Autodesk Inventor part; units mm, degrees
ref_plane "YZ Plane" through (0, 0, 0) normal (1, 0, 0) x (0, 1, 0)
ref_plane "XZ Plane" through (0, 0, 0) normal (0, 1, 0) x (-1, 0, 0)
ref_plane "XY Plane" through (0, 0, 0) normal (0, 0, 1) x (1, 0, 0)
sketch "Sketch1" plane through (0, 0, 0) normal (0, 1, 0) x (-1, 0, 0)
  circle A0 centre (0, 0) radius 6.985
  line L0 (6.985, 0) -> (6.985, -21.59)
  line L1 (6.985, -21.59) -> (-6.985, -21.59)
  line L2 (-6.985, -21.59) -> (-6.985, 0)
  line L3 (0, 0) -> (1.651, 0)
  line L4 (1.651, 0) -> (1.651, -1.651)
  line L5 (1.651, -1.651) -> (-1.651, -1.651)
  line L6 (-1.651, -1.651) -> (-1.651, 1.651)
  line L7 (-1.651, 1.651) -> (1.651, 1.651)
  line L8 (1.651, 1.651) -> (1.651, 0)
  dimension "d0" = 13.97
  dimension "d1" = 21.59
  dimension "d2" = 13.97
  dimension "d3" = 1.651
  dimension "d4" = 1.651
  dimension "d5" = 3.302
  dimension "d6" = 3.302
  dimension "d7" = 3.302
extrude "Extrusion1" add sketch "Sketch1" along normal blind 3.175
sketch "Sketch2" plane through (6.985, 0, -21.59) normal (0, 0, -1) x (-1, 0, 0)
  line L0 (13.97, 3.175) -> (0, 3.175)
  line L1 (6.985, 3.175) -> (-15.875, 3.175)
  line L2 (-15.875, 3.175) -> (-15.875, -19.685)
  line L3 (-15.875, -19.685) -> (29.845, -19.685)
  line L4 (29.845, -19.685) -> (29.845, 3.175)
  line L5 (29.845, 3.175) -> (6.985, 3.175)
  point P0 (6.985, 0)
  dimension "d10" = 22.86
  dimension "d11" = 22.86
  dimension "d12" = 45.72
extrude "Extrusion2" add sketch "Sketch2" along normal blind 3.175
sketch "Sketch3" plane through (6.985, 0, -24.765) normal (0, 0, -1) x (-1, 0, 0)
  line L0 (29.845, 3.175) -> (27.305, 3.175)
  line L1 (29.845, 3.175) -> (-15.875, 3.175)
  line L2 (27.305, 3.175) -> (27.305, 0.635)
  circle A0 centre (27.305, 0.635) radius 1.5875
  line L3 (-15.875, -19.685) -> (-13.335, -19.685)
  line L4 (-13.335, -19.685) -> (-13.335, -17.145)
  circle A1 centre (-13.335, -17.145) radius 1.5875
  point P0 (6.985, 0)
  dimension "d15" = 2.54
  dimension "d16" = 2.54
  dimension "d17" = 3.175
  dimension "d18" = 2.54
  dimension "d19" = 2.54
  dimension "d20" = 3.175
extrude "Extrusion3" cut sketch "Sketch3" against normal blind 3.175
properties part number "Autonomous - Ultrasonic to Servo"
For this review, take the finished solid that the model builds, in its own axes (mm). A direction names the side the tool comes from. Round coordinates to 2 decimals unless told otherwise and drop trailing zeros. Order: outer loops, then holes, each group sorted by start corner. A loop starts at its lowest first (then second) coordinate and runs counter-clockwise, first axis right, second up. Notation, with made-up numbers: (69.25, 45.5) -> (103.25, 45.5) arc R29 ccw to (103.25, 84.5) -> close; hole circle Ø7 at (49.25, 80). An arc over 180 degrees is marked (long way). Write item = value, one per line. Start each with the question number.
1) Take a section at D-D on y = -11.25. State the section outline as (x, z) points (3 decimals), plus the area to 3 significant figures.
2) Take a section at B-B on x = -20.32. State the section outline as (y, z) points (1 decimal), plus the area to 3 significant figures.
3) Take a section at A-A on x = 0. State the section outline as (y, z) points (3 decimals), plus the area to 3 significant figures.
4) Tool access review of faces 1 (the face through (6.985, 2, -11)), 2 (the face through (-1.651, 2, 0)), 3 (the face through (0, 0, -7)): name each direction out of +Z, -Z, +X, -X, +Y, -Y from which nothing blocks a thin tool from reaching the whole face with its end or side.
5) Insertion check: pin 1 (3.5 mm diameter, centred on y = 1, z = 0, fed in from +X) (3 decimals); pin 2 (7 mm diameter, centred on x = -11.5, y = -12, fed in from +Z); pin 3 (12 mm diameter, centred on x = -4, y = -4.5, fed in from +Z); pin 4 (1 mm diameter, centred on y = 2, z = 1, fed in from -X). Each pin has a flat end and moves straight along its axis. Give the tip position at first contact, or say it passes through.
6) Take a section at C-C on z = -6.5. State the section outline as (x, y) points (3 decimals), plus the area to 3 significant figures.
7) The part is to be moulded in two halves that separate along Z. For faces 4 (the face through (1.651, 2, 0)), 5 (the face through (-22.86, -8, -23)), 6 (the face through (0, -8, -24.765)), say which applies: +Z half, -Z half, draft (parallel to the pull), parting line (faces both ways), or undercut.
8) To check wall thickness, follow line 1 (Y direction, x = 20.32, z = -23) (1 decimal); line 2 (Z direction, x = 7, y = -12.5) (3 decimals); line 3 (Y direction, x = -20.32, z = -23.4) (1 decimal). State the ranges of each line that lie inside material, in increasing order. Write a range as from..to.
Verdict:
q1.outline = (-22.86, -24.765) -> (22.86, -24.765) -> (22.86, -21.59) -> (-22.86, -21.59) -> close
q1.area = 145 mm2
q2.outline = (-19.7, -24.8) -> (-1, -24.8) -> (-1, -21.6) -> (-19.7, -21.6) -> close; (2.2, -24.8) -> (3.2, -24.8) -> (3.2, -21.6) -> (2.2, -21.6) -> close
q2.area = 62.5 mm2
q3.outline = (-19.685, -24.765) -> (3.175, -24.765) -> (3.175, -1.651) -> (0, -1.651) -> (0, -21.59) -> (-19.685, -21.59) -> close; (0, 1.651) -> (3.175, 1.651) -> (3.175, 6.985) -> (0, 6.985) -> close
q3.area = 153 mm2
q4.face_1 = +Z, +X, +Y, -Y
q4.face_2 = +Y, -Y
q4.face_3 = +Z, +X, -X, -Y
q5.pin_1 = 6.985
q5.pin_2 = -21.59
q5.pin_3 = 6.98
q5.pin_4 = -6.97
q6.outline = (-6.985, 0) -> (6.985, 0) -> (6.985, 3.175) -> (-6.985, 3.175) -> close
q6.area = 44.4 mm2
q7.face_4 = undercut
q7.face_5 = draft
q7.face_6 = -Z half
q8.line_1 = -19.7..-18.7, -15.6..3.2
q8.line_2 = -24.765..-21.59
q8.line_3 = -19.7..-1, 2.2..3.2
